For this review, take the finished solid that the model builds, in its own axes (mm). A direction names the side the tool comes from. Coordinates: 2 decimals unless noted, no trailing zeros. Order: outer loops, then holes, each group sorted by start corner. A loop starts at its lowest first (then second) coordinate and runs counter-clockwise, first axis right, second up. Notation, with made-up numbers: (-7, -38.5) -> (29, -38.5) arc R13 ccw to (29, -16.5) -> close; hole circle Ø6 at (29.25, 38.25). An arc over 180 degrees is marked (long way). Return JSON: item names as keys, results as strings. Group by question number.
Item 1: Draft analysis for pull direction Y (two halves, no side actions). For faces 1 (the flat face through (0, -4.25, -5)), 2 (the flat face through (-6, 4, 17.8)), 3 (the flat face through (0, 12.75, -5)), state which applies: +Y half, -Y half, draft (parallel to the pull), parting line (faces both ways), or undercut.
Item 2: Take a section at B-B (x = 7). Write out the cut boundary in (y, z), then the cut area to 3 significant figures.
Item 3: Machinability: for faces 4 (the flat face through (0, 11.75, -5)), 5 (the flat face through (0, -5.25, -5)), 6 (the flat face through (3.15, -5, -5)), 7 (the cylindrical face through (-1.27, 5.71, 22.14)), 8 (the flat face through (-3.15, 12, -5)), which of the approach directions +Z, -Z, +X, -X, +Y, -Y give a long, thin tool a straight path to every point of the face, cutting with its end or side? Answer none if there is none.
Item 4: For line 1 along Y through (x, z) = (-2.25, -5.5); line 2 along Z through (x, y) = (3, -15); line 3 along Z through (x, y) = (0.75, -5), list the stretches that pass through material, from the lowest coordinate up.
Item 5: Take a section at A-A (z = -1). Write out the cut boundary in (x, y).
Item 6: Take a section at C-C (z = 34.5). Write out the cut boundary in (x, y), then the cut area to 3 significant figures.
Item 7: Insertion check: pin 1 (3 mm diameter, centred on x = -4.5, y = -10.5, fed in from +Z); pin 2 (1 mm diameter, centred on y = 2.5, z = 24, fed in from +X); pin 3 (1.1 mm diameter, centred on y = 12, z = -6, fed in from +X). Each pin has a flat end and moves straight along its axis. Give the tip position at first contact, or say it passes through.
Autodesk Inventor part; units mm, degrees
ref_plane "YZ Plane" through (0, 0, 0) normal (1, 0, 0) x (0, 1, 0)
ref_plane "XZ Plane" through (0, 0, 0) normal (0, 1, 0) x (-1, 0, 0)
ref_plane "XY Plane" through (0, 0, 0) normal (0, 0, 1) x (1, 0, 0)
sketch "Sketch1" plane through (0, 0, 0) normal (0, 0, 1) x (1, 0, 0)
  line L0 (-8.1, -17.75) -> (8.1, -17.75)
  line L1 (8.1, -17.75) -> (8.1, 17.75)
  line L2 (8.1, 17.75) -> (-8.1, 17.75)
  line L3 (-8.1, 17.75) -> (-8.1, -17.75)
  line L4 (-8.1, -17.75) -> (8.1, 17.75) construction
  line L5 (8.1, -17.75) -> (-8.1, 17.75) construction
  point P0 (0, 0)
  dimension "d0" = 16.2
  dimension "d1" = 35.5
extrude "Extrusion1" add sketch "Sketch1" along normal blind 17.8
sketch "Sketch2" plane through (0, 0, 17.8) normal (0, 0, 1) x (1, 0, 0)
  circle A0 centre (0, 0) radius 5.85
  dimension "d4" = 11.7
extrude "Extrusion2" add sketch "Sketch2" along normal blind 8.8
sketch "Sketch3" plane through (0, 0, 26.6) normal (0, 0, 1) x (1, 0, 0)
  circle A0 centre (0, 0) radius 3
  dimension "d7" = 6
extrude "Extrusion3" add sketch "Sketch3" along normal blind 16
fillet "Fillet1" radius 2 1 edges at (-3, 0, 42.6)
sketch "Sketch4" plane through (0, 0, 0) normal (0, 0, -1) x (-1, 0, 0)
  line L0 (-3.15, 12.75) -> (3.15, 12.75)
  line L1 (3.15, 12.75) -> (3.15, 11.75)
  line L2 (3.15, 11.75) -> (-3.15, 11.75)
  line L3 (-3.15, 11.75) -> (-3.15, 12.75)
  line L4 (-3.15, 12.75) -> (3.15, 11.75) construction
  line L5 (3.15, 12.75) -> (-3.15, 11.75) construction
  line L6 (-3.15, -4.25) -> (3.15, -4.25)
  line L7 (3.15, -4.25) -> (3.15, -5.25)
  line L8 (3.15, -5.25) -> (-3.15, -5.25)
  line L9 (-3.15, -5.25) -> (-3.15, -4.25)
  line L10 (-3.15, -4.25) -> (3.15, -5.25) construction
  line L11 (3.15, -4.25) -> (-3.15, -5.25) construction
  line L12 (-8.1, 17.75) -> (8.1, 17.75)
  line L13 (8.1, -17.75) -> (-8.1, -17.75)
  point P0 (0, 0)
  point P1 (0, 12.25)
  point P2 (0, -4.75)
  point P3 (0, 12.25)
  point P4 (0, -4.75)
  dimension "d11" = 6.3
  dimension "d12" = 1
  dimension "d13" = 6.3
  dimension "d14" = 1
  dimension "d15" = 5
  dimension "d16" = 12.5
extrude "Extrusion4" add sketch "Sketch4" along normal blind 10
thread "Thread1"
properties part number "Schalter"
Findings below:
{
 "1": {"face 1": "undercut", "face 2": "draft", "face 3": "+Y half"},
 "2": {"outline": "(-17.75, 0) -> (17.75, 0) -> (17.75, 17.8) -> (-17.75, 17.8) -> close", "area": "632 mm2"},
 "3": {"face 4": "-Z, +X, -X", "face 5": "-Z, +X, -X, -Y", "face 6": "-Z, +X, +Y, -Y", "face 7": "+Z", "face 8": "-Z, -X, +Y, -Y"},
 "4": {"line 1": "y = -5.25 to -4.25, 11.75 to 12.75", "line 2": "z = 0 to 17.8", "line 3": "z = -10 to 26.6"},
 "5": {"outline": "(-3.15, -5.25) -> (3.15, -5.25) -> (3.15, -4.25) -> (-3.15, -4.25) -> close; (-3.15, 11.75) -> (3.15, 11.75) -> (3.15, 12.75) -> (-3.15, 12.75) -> close"},
 "6": {"outline": "circle Ø6 at (0, 0)", "area": "28.3 mm2"},
 "7": {"pin 1": "stops at z = 17.8", "pin 2": "stops at x = 5.5", "pin 3": "stops at x = 3.15"}
}
